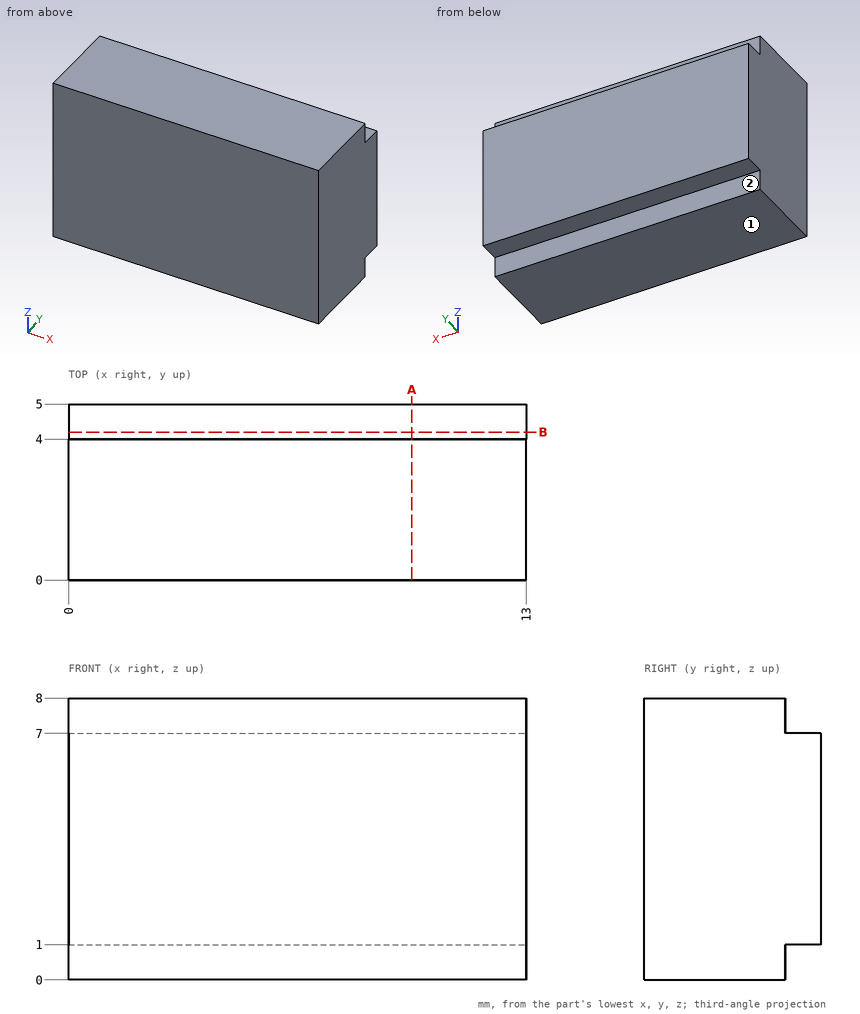
Design review of the part shown in the three views and the two pictorial views. Dimensions are in mm from the part's minimum x, y and z. A direction names the side the tool comes from. Coordinates: 2 decimals unless noted, no trailing zeros. Order: outer loops, then holes, each group sorted by start corner. A loop starts at its lowest first (then second) coordinate and runs counter-clockwise, first axis right, second up.
1) For the marked faces 1 and 2, list the 3-axis set-ups (+Z, -Z, +X, -X, +Y, -Y) from which the entire face can be reached by the end or side of a thin tool; tool diameter is ignored.
2) Take a section at A-A, the plane x = 9.75. Give the boundary of the cut face in (y, z), and give its area (3 significant figures).
3) Take a section at B-B, the plane y = 4.2. Give the boundary of the cut face in (x, z).
4) Wall thickness on line 1 along Y through (x, z) = (9, 0.5); line 2 along Z through (x, y) = (12, 4.4): over which ranges is each line inside the solid? List them lowest first.
Returned:
1. face 1: -Z, +X, -X, +Y, -Y
1. face 2: -Z, +X, -X, +Y
2. outline: (0, 0) - (4, 0) - (4, 1) - (5, 1) - (5, 7) - (4, 7) - (4, 8) - (0, 8) - close
2. area: 38.0 mm2
3. outline: (0, 1) - (13, 1) - (13, 7) - (0, 7) - close
4. line 1: y = 0 to 4
4. line 2: z = 1 to 7
